Build history of the part. All positions in model axes, mm. A direction names the side the tool comes from. Give positions to 0.01 mm unless a question says otherwise; leave off trailing zeros. Loops run counter-clockwise (first coordinate to the right, second up) from the corner with the lowest first, then second, coordinate; pieces in that order, holes last. Notation, with made-up numbers: M -7,53 L 19,53 A20 cw 19,68 Z; hole C -32.5,-30.5 d11. An arc over 180 degrees is marked long. Put each result on its own line as item: value.
Autodesk Inventor part; units mm, degrees
ref_plane "YZ Plane" through (0, 0, 0) normal (1, 0, 0) x (0, 1, 0)
ref_plane "XZ Plane" through (0, 0, 0) normal (0, 1, 0) x (-1, 0, 0)
ref_plane "XY Plane" through (0, 0, 0) normal (0, 0, 1) x (1, 0, 0)
sketch "Esboço4" plane through (0, 0, 0) normal (0, 1, 0) x (-1, 0, 0)
  line L0 (0, -15) -> (0, -135)
  line L1 (-15, -150) -> (-55, -150)
  line L2 (-70, -135) -> (-70, -15)
  line L3 (-55, 0) -> (-15, 0)
  arc A0 (-15, -150) -> (0, -135) centre (-15, -135) ccw
  arc A1 (-70, -135) -> (-55, -150) centre (-55, -135) ccw
  arc A2 (-55, 0) -> (-70, -15) centre (-55, -15) ccw
  arc A3 (0, -15) -> (-15, 0) centre (-15, -15) ccw
  point P0 (0, 0)
  point P1 (0, -150)
  point P2 (-70, -150)
  dimension "d7" = 150
  dimension "d8" = 70
  dimension "d9" = 15
extrude "Extrusão2" add sketch "Esboço4" along normal blind 8
sketch "Esboço5" plane through (0, 8, 0) normal (0, 1, 0) x (1, 0, 0)
  line L0 (15, 0) -> (55, 0)
  line L1 (55, 150) -> (15, 150)
  circle A0 centre (35, 61) radius 2.5
  circle A1 centre (35, 68) radius 2.5
  point P0 (0, 0)
extrude "Extrusão3" cut sketch "Esboço5" against normal through all
sketch "Sketch7" plane through (0, 0, 0) normal (0, -1, 0) x (1, 0, 0)
  circle A0 centre (35, -61) radius 2
  circle A1 centre (35, -68) radius 2
  line L0 (43, -68) -> (43, -74.75)
  line L1 (43, -74.75) -> (27, -74.75)
  line L2 (27, -74.75) -> (27, -54.25)
  line L3 (27, -54.25) -> (43, -54.25)
  line L4 (43, -54.25) -> (43, -68)
  point P0 (0, 0)
  dimension "d25" = 8
extrude "Extrusion4" add sketch "Sketch7" along normal blind 10
fillet "Fillet4" radius 2 8 edges at (43, -5, -54.25) (43, -5, -74.75) (43, -10, -64.5) (35, -10, -54.25) (27, -10, -64.5) (35, -10, -74.75) (27, -5, -74.75) (27, -5, -54.25)
fillet "Fillet5" radius 0.5 2 edges at (32.5, 8, -61) (32.5, 8, -68)
properties part number "Base superior(suporte)" material "ABS plástico"
Q1. Drop flat-ended pins along their axis: pin 1 Ø1.5 at (y, z) = (-2.5, -102.5) entering from -X; pin 2 Ø3 at (y, z) = (-6.5, -73) entering from -X; pin 3 Ø1.5 at (x, y) = (23, 1) entering from +Z; pin 4 Ø8 at (x, z) = (46.5, -108.5) entering from -Y. Give the stop position or say it passes through.
Here are the results:
pin 1: through
pin 2: x = 27
pin 3: z = 0
pin 4: y = 0
Q2. Tool access for faces 1 (the flat face through (35, -4, -74.75)), 2 (the flat face through (43, -4, -64)), 3 (the flat face through (27, -4, -65)), 4 (the cylindrical face through (36.075, -4.93, -69.686)), 5 (the cylindrical face through (37.31, 3.8, -60.04)): list every direction of +Z, -Z, +X, -X, +Y, -Y with a clear straight run to the whole face (end or side of a thin tool).
Here are the results:
face 1: -Z, +X, -X, -Y
face 2: +Z, -Z, +X, -Y
face 3: +Z, -Z, -X, -Y
face 4: +Y, -Y
face 5: +Y
Q3. Slice it at C-C (y = 2.5). List the corners of the cut face in (x, z).
Here are the results:
outline: M 0,-135 A15 ccw 15,-150 L 55,-150 A15 ccw 70,-135 L 70,-15 A15 ccw 55,0 L 15,0 A15 ccw 0,-15 Z; hole C 35,-68 d5; hole C 35,-61 d5
Q4. Probe line 1 (Z direction, x = 35, y = 2); line 2 (Z direction, x = 35, y = -5.75); line 3 (X direction, y = 2.25, z = -61). List the from-to ranges inside material, lowest first. Write a range as from..to.
Here are the results:
line 1: -150..-70.5, -65.5..-63.5, -58.5..0
line 2: -74.75..-70, -66..-63, -59..-54.25
line 3: 0..32.5, 37.5..70
Q5. Slice it at A-A (x = 35). State how many separate pieces and enclosed holes the cut face has, and give its area (3 significant figures).
Here are the results:
separate pieces: 3
enclosed holes: 0
area: 1,240 mm²
Q6. Slice it at B-B (z = -61). List the corners of the cut face in (x, y), and give its area (3 significant figures).
Here are the results:
outline: M 0,0 L 27,0 L 27,-8 A2 ccw 29,-10 L 33,-10 L 33,0 L 32.5,0 L 32.5,7.5 A0.5 ccw 32,8 L 0,8 Z; M 37,-10 L 41,-10 A2 ccw 43,-8 L 43,0 L 70,0 L 70,8 L 38,8 A0.5 ccw 37.5,7.5 L 37.5,0 L 37,0 Z
area: 638 mm²
Q7. Mould opens along X. For faces 6 (the cylindrical face through (4.51, 3.94, -4.28)), 7 (the cylindrical face through (37.31, 3.8, -67.04)), 8 (the flat face through (35, -4, -54.25)) say: pulls with the +X half, pulls with the -X half, needs draft (parallel to the pull), parting line crosses it, or undercut.
Here are the results:
face 6: pulls with the -X half
face 7: undercut
face 8: needs draft
Q8. Slice it at D-D (x = 16.5). List the corners of the cut face in (y, z).
Here are the results:
outline: M 0,-150 L 8,-150 L 8,0 L 0,0 Z
